```python
from build123d import *

# Parameters (mm, degrees)
SKETCH_1_R                   = 9.75
EXTRUDE_1_DEPTH              = 19.4
SKETCH_1_3_R                 = 9.75
EXTRUDE_2_DEPTH              = 29.4
SKETCH_2_R                   = 5
CUT_EXTRUDE_1_DEPTH          = 69.371576697
FILLET_1_R                   = 80
HOLE_WIZARD_M8_1_D           = 9
HOLE_WIZARD_M8_1_CBORE_D     = 15
HOLE_WIZARD_M8_1_CBORE_DEPTH = 8


with BuildPart() as part:
    # 스케치1 → 보스-돌출1 (new body)
    with BuildSketch(Plane.XY):
        with Locations((-50.75, 0)):
            Circle(SKETCH_1_R)
        with BuildLine():
            Line((-51.227471847, -9.738301733), (0, -12.25))
            Line((0, -12.25), (0, 12.25))
            Line((0, 12.25), (-51.227471847, 9.738301733))
            ThreePointArc((-51.227471847, 9.738301733), (-44.026639624, 7.061085274), (-41, 0))
            ThreePointArc((-41, 0), (-44.026639624, -7.061085274), (-51.227471847, -9.738301733))
        make_face()
        with BuildLine():
            Line((0, 12.25), (0, -12.25))
            Line((0, -12.25), (51.227471847, -9.738301733))
            ThreePointArc((51.227471847, -9.738301733), (41, 0), (51.227471847, 9.738301733))
            Line((51.227471847, 9.738301733), (0, 12.25))
        make_face()
        with Locations((50.75, 0)):
            Circle(SKETCH_1_R)
    extrude(amount=EXTRUDE_1_DEPTH)

    # 스케치1<3> → 보스-돌출2 (add)
    with BuildSketch(Plane.XY):
        with Locations(Location((-50.75, 0, 0), (0, 0, 92.806981348))):
            Circle(SKETCH_1_3_R)
        with Locations(Location((50.75, 0, 0), (0, 0, 87.193018652))):
            Circle(SKETCH_1_3_R)
    extrude(amount=EXTRUDE_2_DEPTH)

    # 스케치2 → 컷-돌출1 (cut, through all)
    with BuildSketch(Plane.XY):
        Circle(SKETCH_2_R)
    extrude(amount=CUT_EXTRUDE_1_DEPTH, mode=Mode.SUBTRACT)

    # 필렛1
    # the kernel refuses this fillet: 80 mm, written as the material it takes off along each edge
    with BuildSketch(Plane(origin=(0, 12.25, -9.806059822), x_dir=(0.9988001777044758, -0.048971471465613654, 0), z_dir=(0, 0, 1))) as fillet_1_piece_1:
        with BuildLine():
            CenterArc((FILLET_1_R * 0.0490302991116, -FILLET_1_R), FILLET_1_R, 90, 5.613962695)
            Line((-FILLET_1_R * 0.048795129693, -FILLET_1_R * 0.00479641003501), (0, 0))
            Line((0, 0), (FILLET_1_R * 0.0490302991116, 0))
        make_face()
    extrude(amount=39.012119645, mode=Mode.SUBTRACT)
    with BuildSketch(Plane(origin=(0, -12.25, -9.806059822), x_dir=(0.9988001777044758, 0.0489714714656137, 0), z_dir=(0, 0, 1))) as fillet_1_piece_2:
        with BuildLine():
            CenterArc((FILLET_1_R * 0.0490302991116, FILLET_1_R), FILLET_1_R, 264.386037305, 5.613962695)
            Line((-FILLET_1_R * 0.048795129693, FILLET_1_R * 0.00479641003501), (0, 0))
            Line((0, 0), (FILLET_1_R * 0.0490302991116, 0))
        make_face()
    extrude(amount=39.012119645, mode=Mode.SUBTRACT)

    # M8 소켓 머리 캡 나사용 카운터보어1 (through all)
    with Locations(Plane(origin=(0, 0, 0), x_dir=(-1, 0, 0), z_dir=(0, 0, -1))):
        with Locations((-50.75, 0), (50.75, 0)):
            CounterBoreHole(HOLE_WIZARD_M8_1_D / 2, HOLE_WIZARD_M8_1_CBORE_D / 2, HOLE_WIZARD_M8_1_CBORE_DEPTH)


solid = part.part
```
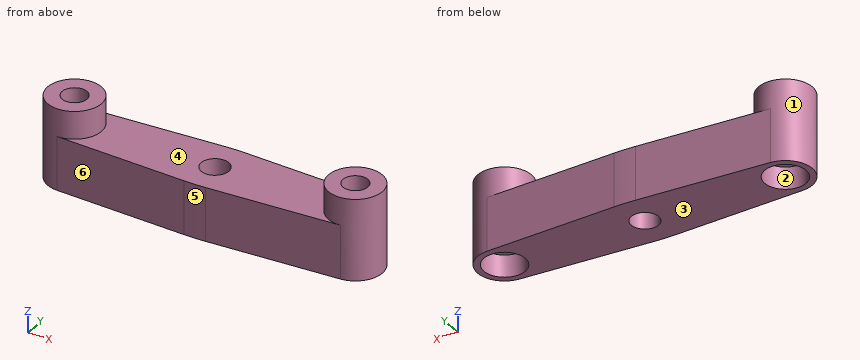
Read the model definition and answer for the solid it produces. Units are mm, in the model's axes. Face numbers are marked on the shaded views. A direction names the side the tool comes from. Round coordinates to 2 decimals unless told otherwise and drop trailing zeros. Write each loop counter-clockwise with the first axis right and the second up, starting at its lowest first coordinate (ties: lowest second). Pieces come first, ordered by that corner, then holes. Notation, with made-up numbers: (-2.75, 0) -> (10.25, 0) arc R19 cw to (10.25, 32) -> close; hole circle Ø2 at (19, 58.5). An arc over 180 degrees is marked (long way). Answer in a Markdown table with one row per item. Add a question column.
1) Given P1, Ø4, axis at x = 19.5, z = 22, coming from the +Y side; P2, Ø12, axis at x = 9, y = -2.5, coming from the +Z side; P3, Ø12, axis at y = -1, z = 14, coming from the +X side; P4, Ø12, axis at x = -50.75, y = 0, coming from the -Z side, each flat-ended and moving along its own axis, determine where each tip first touches the part or whether it passes through.
2) Determine the mould class of the marked faces 4, 5 and 6 for opening direction X: pulls with the +X half, pulls with the -X half, needs draft (parallel to the pull), parting line crosses it, or undercut.
3) Find section D-D, the plane z = 22.5. Determine the outline of the cut face in (x, y).
4) Consider line 1 (Y direction, x = 50.75, z = 14.25); line 2 (X direction, y = -3.5, z = 10.5); line 3 (X direction, y = 5.5, z = 3). Determine where each line is inside the solid, lowest interval first.
5) Find section A-A, the plane x = 0. Determine the outline of the cut face in (y, z).
6) Find section C-C, the plane y = -1.5. Determine the outline of the cut face in (x, z).
7) Which of the six approach directions +Z, -Z, +X, -X, +Y, -Y give full straight-line access (tool end or side, diameter ignored) to the marked faces 1, 2 and 3?
8) Find section B-B, the plane z = 2. Determine the outline of the cut face in (x, y), and give its area (3 significant figures).
Findings below:
| question | item | result |
|---|---|---|
| 1 | P1 | through |
| 1 | P2 | z = 19.4 |
| 1 | P3 | x = 60.5 |
| 1 | P4 | z = 8 |
| 2 | face 4 | undercut |
| 2 | face 5 | parting line crosses it |
| 2 | face 6 | pulls with the -X half |
| 3 | outline | circle Ø19.5 at (-50.75, 0); circle Ø19.5 at (50.75, 0); hole circle Ø9 at (-50.75, 0); hole circle Ø9 at (50.75, 0) |
| 4 | line 1 | -9.76 to -4.5, 4.5 to 9.76 |
| 4 | line 2 | -59.85 to -53.58, -47.92 to -3.57, 3.57 to 47.92, 53.58 to 59.85 |
| 4 | line 3 | -58.8 to -55.85, -45.65 to 45.65, 55.85 to 58.8 |
| 5 | outline | (-12.15, 0) -> (-5, 0) -> (-5, 19.4) -> (-12.15, 19.4) -> close; (5, 0) -> (12.15, 0) -> (12.15, 19.4) -> (5, 19.4) -> close |
| 6 | outline | (-60.38, 0) -> (-58.1, 0) -> (-58.1, 8) -> (-54.99, 8) -> (-54.99, 29.4) -> (-60.38, 29.4) -> close; (-46.51, 8) -> (-43.4, 8) -> (-43.4, 0) -> (-4.77, 0) -> (-4.77, 19.4) -> (-41.12, 19.4) -> (-41.12, 29.4) -> (-46.51, 29.4) -> close; (4.77, 0) -> (43.4, 0) -> (43.4, 8) -> (46.51, 8) -> (46.51, 29.4) -> (41.12, 29.4) -> (41.12, 19.4) -> (4.77, 19.4) -> close; (54.99, 8) -> (58.1, 8) -> (58.1, 0) -> (60.38, 0) -> (60.38, 29.4) -> (54.99, 29.4) -> close |
| 7 | face 1 | +Z |
| 7 | face 2 | -Z |
| 7 | face 3 | -Z, +X, -X, +Y, -Y |
| 8 | outline | (-51.23, -9.74) -> (-3.92, -12.06) arc R80 ccw to (3.92, -12.06) -> (51.23, -9.74) arc R9.75 ccw to (51.23, 9.74) -> (3.92, 12.06) arc R80 ccw to (-3.92, 12.06) -> (-51.23, 9.74) arc R9.75 ccw to start; hole circle Ø15 at (-50.75, 0); hole circle Ø10 at (0, 0); hole circle Ø15 at (50.75, 0) |
| 8 | area | 2,100 mm² |
